Input: dimensioned drawing with shaded views. Units: mm. Origin: part minimum x, y, z. Round coordinates to 2 decimals unless told otherwise and drop trailing zeros. Loops run counter-clockwise (first coordinate to the right, second up) from the corner with the lowest first, then second, coordinate; pieces in that order, holes last. Notation, with made-up numbers: M 4,28 L 44,28 A8 cw 44,41 Z; hole C -29.75,56.25 d10. An arc over 180 degrees is marked long. Answer as a JSON object with one key per item and string values.
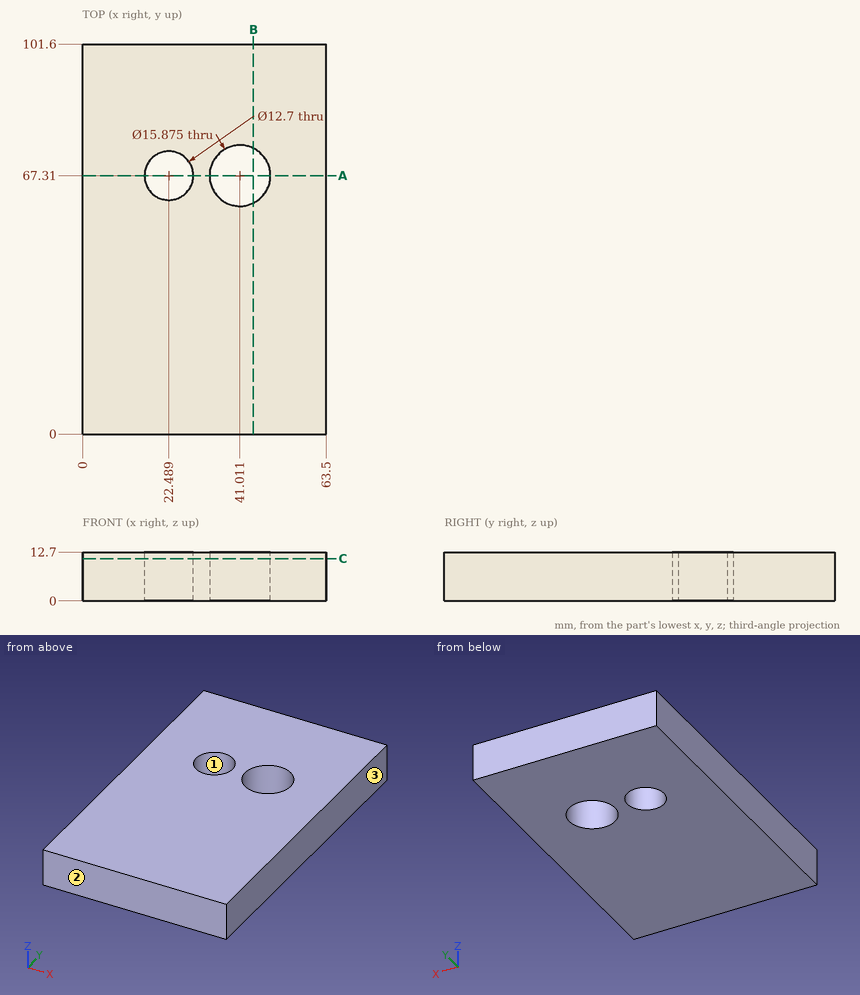
Item 1: Line query: probe 1 along X at (y, z) = (66, 2.5); probe 2 along X at (y, z) = (63, 3.5) (1 decimal); probe 3 along Y at (x, z) = (23, 10). Output: solid intervals per line, ascending. Write a range as from..to.
Answer sheet:
{"probe 1": "x = 0..16.28, 28.7..33.18, 48.84..63.5", "probe 2": "x = 0..17.8, 27.2..34.3, 47.7..63.5", "probe 3": "y = 0..60.98, 73.64..101.6"}
Item 2: Section C-C on z = 11. Give the number of separate pieces and of enclosed holes in the cut face, then the cut area to 3 significant figures.
Answer sheet:
{"separate pieces": "1", "enclosed holes": "2", "area": "6,130 mm²"}
Item 3: Pull-direction query (Y, two-part tool) for the marked faces 1, 2 and 3; classes: pulls with the +Y half, pulls with the -Y half, needs draft (parallel to the pull), parting line crosses it, or undercut.
Answer sheet:
{"face 1": "undercut", "face 2": "pulls with the -Y half", "face 3": "needs draft"}
Item 4: Section B-B on x = 44.5. Return the cut outline in (y, z), then the cut area to 3 significant figures.
Answer sheet:
{"outline": "M 0,0 L 60.18,0 L 60.18,12.7 L 0,12.7 Z; M 74.44,0 L 101.6,0 L 101.6,12.7 L 74.44,12.7 Z", "area": "1,110 mm²"}
Item 5: Section A-A on y = 67.31. Return the cut outline in (x, z).
Answer sheet:
{"outline": "M 0,0 L 16.14,0 L 16.14,12.7 L 0,12.7 Z; M 28.84,0 L 33.07,0 L 33.07,12.7 L 28.84,12.7 Z; M 48.95,0 L 63.5,0 L 63.5,12.7 L 48.95,12.7 Z"}
